For this review, use the dimensioned drawing (mm, ordinates from the lowest corner) and the shaded views. A direction names the side the tool comes from. Round coordinates to 2 decimals unless told otherwise and drop trailing zeros. Order: outer loops, then holes, each group sorted by start corner. A loop starts at its lowest first (then second) coordinate and runs counter-clockwise, first axis right, second up. Notation, with made-up numbers: M -17.5,-32 L 34.5,-32 A26 cw 34.5,2 Z; hole C 50.5,56.25 d3. An arc over 180 degrees is marked long. Use a Markdown table: item, result. Add a question column.
1. Consider section B-B on y = 25.4. State the section outline as (x, z) points, then the cut area to 3 significant figures.
2. Consider section C-C on z = 9.75. State the section outline as (x, y) points, then the cut area to 3 significant figures.
3. Insertion check: P1, Ø6, axis at x = 41, z = 9.5, coming from the -Y side (1 decimal); P2, Ø1, axis at x = 13, y = 8.5, coming from the +Z side; P3, Ø3, axis at y = 21, z = 14, coming from the -X side. Each pin has a flat end and moves straight along its axis. Give the tip position at first contact, or say it passes through.
4. The part is to be moulded in two halves that separate along Y. For the marked faces 3, 4, 5 and 6, say which applies: +Y half, -Y half, draft (parallel to the pull), parting line (faces both ways), or undercut.
5. Consider section A-A on x = 25.4. State the section outline as (y, z) points.
6. For the marked faces 1 and 2, list the 3-axis set-ups (+Z, -Z, +X, -X, +Y, -Y) from which the entire face can be reached by the end or side of a thin tool; tool diameter is ignored.
7. Consider section D-D on z = 20.5. State the section outline as (x, y) points, then the cut area to 3 significant figures.
8. To check wall thickness, follow probe 1 along Y at (x, z) = (25.4, 7.75); probe 2 along Y at (x, z) = (25.5, 22.25) (1 decimal); probe 3 along X at (y, z) = (35, 23.5). State the ranges of each line that lie inside material, in increasing order.
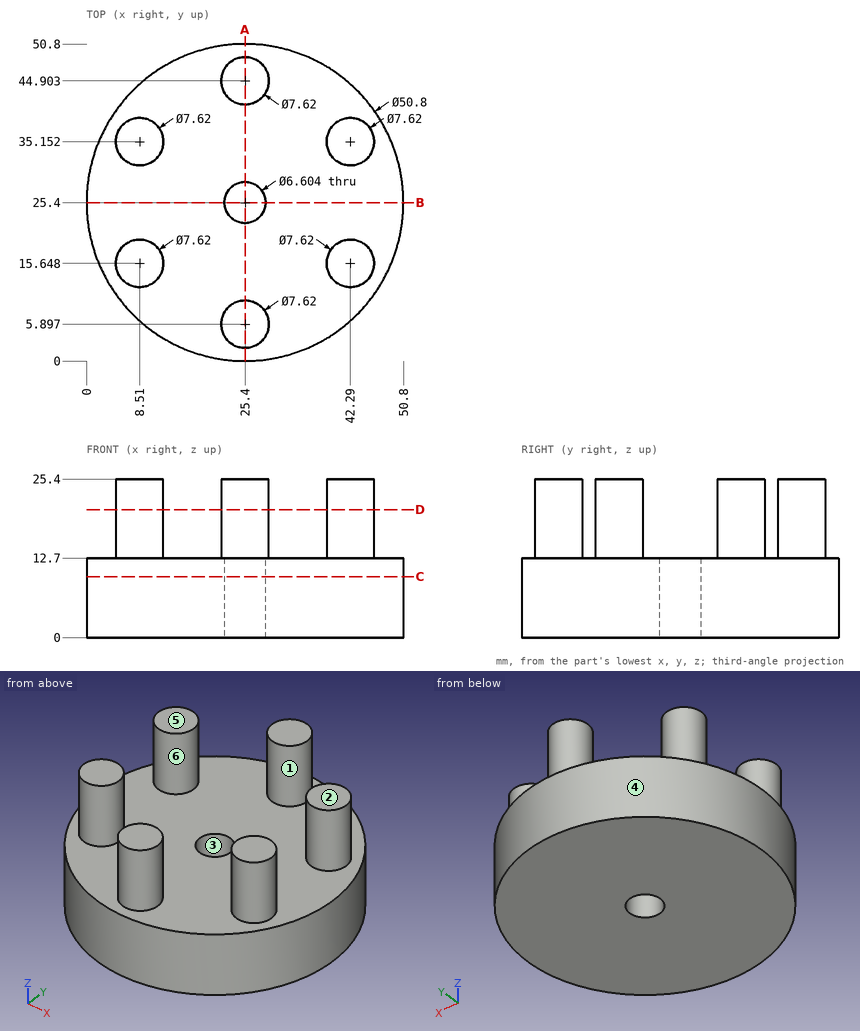
Answer block:
| question | item | result |
|---|---|---|
| 1 | outline | M 0,0 L 22.1,0 L 22.1,12.7 L 0,12.7 Z; M 28.7,0 L 50.8,0 L 50.8,12.7 L 28.7,12.7 Z |
| 1 | area | 561 mm^2 |
| 2 | outline | C 25.4,25.4 d50.8; hole C 25.4,25.4 d6.6 |
| 2 | area | 1,990 mm^2 |
| 3 | P1 | y = 3.3 |
| 3 | P2 | z = 12.7 |
| 3 | P3 | x = 0.26 |
| 4 | face 3 | undercut |
| 4 | face 4 | parting line |
| 4 | face 5 | draft |
| 4 | face 6 | undercut |
| 5 | outline | M 0,0 L 22.1,0 L 22.1,12.7 L 9.71,12.7 L 9.71,25.4 L 2.09,25.4 L 2.09,12.7 L 0,12.7 Z; M 28.7,0 L 50.8,0 L 50.8,12.7 L 48.71,12.7 L 48.71,25.4 L 41.09,25.4 L 41.09,12.7 L 28.7,12.7 Z |
| 6 | face 1 | +Z |
| 6 | face 2 | +Z, +X, -X, +Y, -Y |
| 7 | outline | C 8.51,15.65 d7.62; C 8.51,35.15 d7.62; C 25.4,5.9 d7.62; C 25.4,44.9 d7.62; C 42.29,15.65 d7.62; C 42.29,35.15 d7.62 |
| 7 | area | 274 mm^2 |
| 8 | probe 1 | 0 to 22.1, 28.7 to 50.8 |
| 8 | probe 2 | 2.1 to 9.7, 41.1 to 48.7 |
| 8 | probe 3 | 4.7 to 12.32, 38.48 to 46.1 |
